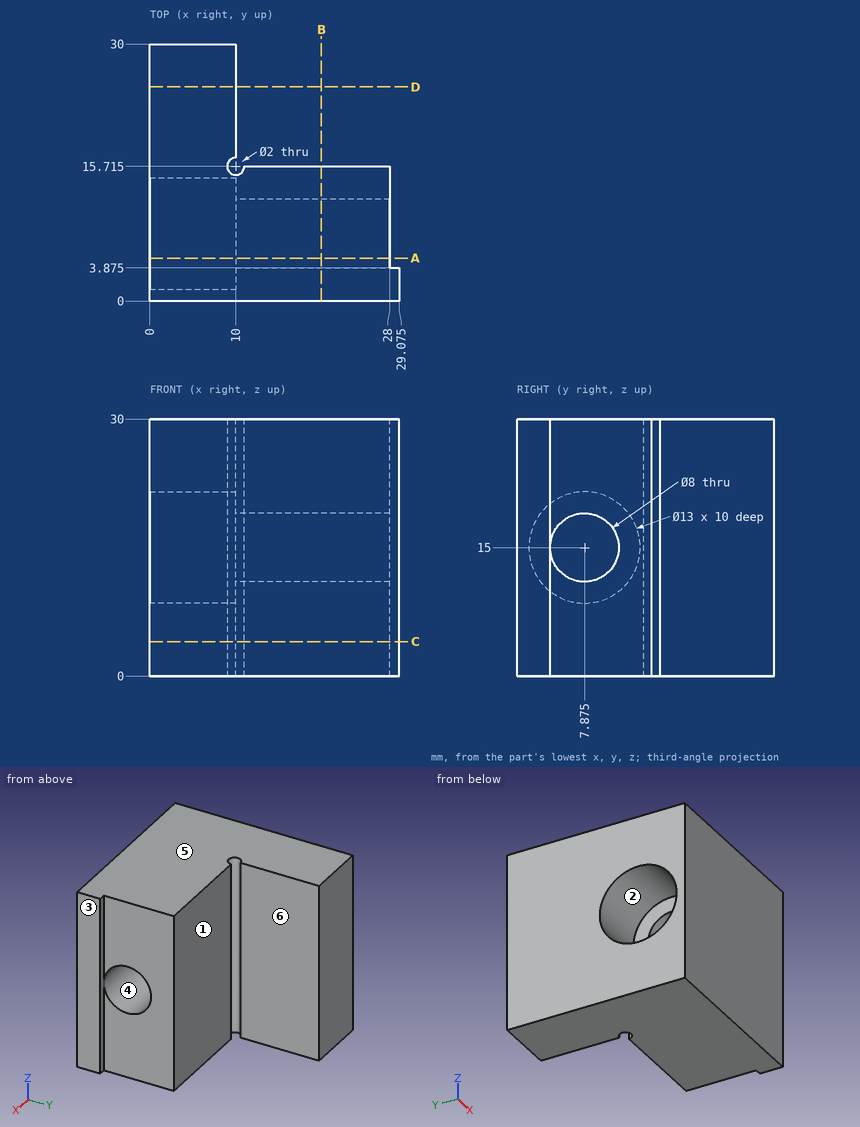
Could you check a few things on this drawing? It's one solid part, dimensions in mm from its lowest x, y, z. A direction names the side the tool comes from. Coordinates: 2 decimals unless noted, no trailing zeros. Order: outer loops, then holes, each group sorted by start corner. A loop starts at its lowest first (then second) coordinate and runs counter-clockwise, first axis right, second up. Notation, with made-up numbers: (-39.75, -27) - (7.25, -27) arc R23 cw to (7.25, 2) - close; hole circle Ø4 at (79.5, -39). An arc over 180 degrees is marked (long way). One line per question, with ' | ' between items. Start each with the question number.
1. If we mould it in two halves opening along Z, with no side actions, what happens to the marked faces 4, 5 and 6? For each: released by +Z, released by -Z, zero draft, split by the parting line, or undercut.
2. If we section it at C-C (z = 4): Write out the boundary of the cut face in (x, y) (1 decimal).
3. If we section it at A-A (y = 5): Write out the boundary of the cut face in (x, z).
4. Which directions (+Z, -Z, +X, -X, +Y, -Y) give clear straight access to the entire face, cutting with the end or side of a thin tool? Please do the marked faces 1, 2 and 3.
5. If we section it at B-B (x = 20): Write out the boundary of the cut face in (y, z) (1 decimal).
6. If we section it at D-D (y = 25): Write out the boundary of the cut face in (x, z).
7. I'm going to push flat-ended pins straight in: pin 1 Ø5 at (y, z) = (7.87, 15) entering from +X; pin 2 Ø8.5 at (x, z) = (15.5, 10.5) entering from +Y (3 decimals); pin 3 Ø6 at (y, z) = (21, 13.5) entering from +X; pin 4 Ø10 at (y, z) = (15.5, 13) entering from +X. Where does each tip first touch, or does it pass through?
8. Please list where these lines run through material, in increasing order: line 1 along X through (y, z) = (13, 12); line 2 along Z through (x, y) = (2.75, 7.5); line 3 along X through (y, z) = (8.5, 3.75). Write a range as [from, to].
Model answer:
1) face 4: undercut | face 5: released by +Z | face 6: zero draft
2) outline: (0, 0) - (29.1, 0) - (29.1, 3.9) - (28, 3.9) - (28, 15.7) - (11, 15.7) arc R1 cw (long way) to (10, 16.7) - (10, 30) - (0, 30) - close
3) outline: (0, 0) - (28, 0) - (28, 12.22) - (10, 12.22) - (10, 9.17) - (0, 9.17) - close; (0, 20.83) - (10, 20.83) - (10, 17.78) - (28, 17.78) - (28, 30) - (0, 30) - close
4) face 1: +Z, -Z, +X, +Y | face 2: -X | face 3: +Z, -Z, +X, +Y, -Y
5) outline: (0, 0) - (15.7, 0) - (15.7, 30) - (0, 30) - close; hole circle Ø8 at (7.9, 15)
6) outline: (0, 0) - (10, 0) - (10, 30) - (0, 30) - close
7) pin 1: passes through | pin 2: stops at y = 15.715 | pin 3: stops at x = 10 | pin 4: stops at x = 28
8) line 1: x = [10, 28] | line 2: z = [0, 8.51], [21.49, 30] | line 3: x = [0, 28]
